```python
from build123d import *

# Parameters (mm, degrees)
F0_W          = 101.6
F0_H          = 101.6
F1_DEPTH      = 101.6
F3_R          = 14.402071
F4_DEPTH      = 25.4
F4_DEPTH_BACK = 127


with BuildPart() as f1:
    # F0 (on Front) → F1 (new body)
    with BuildSketch(Plane.XZ):
        with Locations((50.8, 50.8)):
            Rectangle(F0_W, F0_H)
    extrude(amount=F1_DEPTH)

    # F3 (on offset) → F4 (join, two sides)
    with BuildSketch(Plane.XZ.offset(101.6)) as f4_sk:
        Circle(F3_R)
    extrude(amount=F4_DEPTH)
    extrude(f4_sk.sketch, amount=-F4_DEPTH_BACK)


solid = f1.part
```
For this review, take the finished solid that the model builds, in its own axes (mm). A direction names the side the tool comes from. Give positions to 0.01 mm unless a question says otherwise; leave off trailing zeros. Write each loop counter-clockwise with the first axis right and the second up, starting at its lowest first coordinate (ties: lowest second). Pieces come first, ordered by that corner, then holes. Notation, with made-up numbers: M 4.25,66 L 8.25,66 A22 ccw 8.25,105 Z; hole C -3.75,15 d4. An arc over 180 degrees is marked long. Answer as a JSON object with one key per item and string values. Group by question number.
Item 1: Tool access review of faces 1 (the flat face through (50, -50, 101.6)), 2 (the flat face through (0, -50, 57)), 3 (the flat face through (57, -50, 0)): name each direction out of +Z, -Z, +X, -X, +Y, -Y from which nothing blocks a thin tool from reaching the whole face with its end or side.
Item 2: Consider section C-C on z = 24. Write out the cut boundary in (x, y).
Item 3: Consider section D-D on x = 53. Write out the cut boundary in (y, z).
Item 4: Consider section B-B on y = 4. Write out the cut boundary in (x, z), plus the area to 3 significant figures.
Item 5: Consider section A-A on x = 2. Write out the cut boundary in (y, z), plus the area to 3 significant figures.
Item 6: For pin 1 Ø10 at (x, z) = (20.5, 17) entering from -Y; pin 2 Ø1 at (x, y) = (86.5, -13) entering from -Z; pin 3 Ø8 at (x, z) = (14, 13.5) entering from +Y, all flat-tipped, find the tip position at first contact; note any pin that passes through.
Item 7: For probe 1 along Z at (x, y) = (92.5, -101); probe 2 along Y at (x, z) = (70.5, 16), list the stretches that pass through material, from the lowest coordinate up. Write a range as [from, to].
Check result:
{
 "1": {"face 1": "+Z, +X, -X, +Y, -Y", "face 2": "+Z, -X, +Y, -Y", "face 3": "-Z, +X, +Y, -Y"},
 "2": {"outline": "M 0,-101.6 L 101.6,-101.6 L 101.6,0 L 0,0 Z"},
 "3": {"outline": "M -101.6,0 L 0,0 L 0,101.6 L -101.6,101.6 Z"},
 "4": {"outline": "C 0,0 d28.8", "area": "652 mm^2"},
 "5": {"outline": "M -127,-14.26 L 25.4,-14.26 L 25.4,14.26 L 0,14.26 L 0,101.6 L -101.6,101.6 L -101.6,14.26 L -127,14.26 Z", "area": "13,200 mm^2"},
 "6": {"pin 1": "stops at y = -101.6", "pin 2": "stops at z = 0", "pin 3": "stops at y = 0"},
 "7": {"probe 1": "z = [0, 101.6]", "probe 2": "y = [-101.6, 0]"}
}
